CAD build for the part. Positions are in the model's coordinates, mm. Face numbers are marked on the shaded views. Give positions to 0.01 mm unless a question says otherwise; leave off trailing zeros. Loops run counter-clockwise (first coordinate to the right, second up) from the corner with the lowest first, then second, coordinate; pieces in that order, holes last. Notation, with made-up numbers: (70, 0.5) -> (77, 0.5) arc R21 cw to (77, 30.5) -> close; hole circle Ø3 at (13, 13). An arc over 180 degrees is marked (long way). Use one line per item in the form item = value.
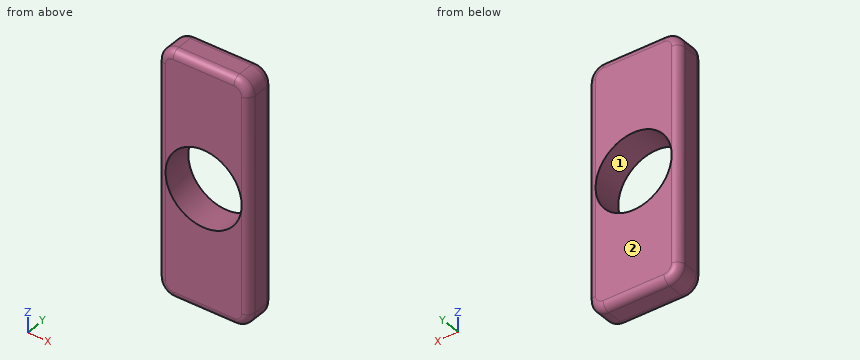
```python
from build123d import *

# Parameters (mm, degrees)
F0_W     = 30
F0_H     = 80
F1_DEPTH = 10
F2_R     = 5
F3_R     = 5
F4_R     = 5
F5_R     = 5
F6_R     = 2.5
F7_R     = 2.5
F9_D     = 25


with BuildPart() as f1:
    # F0 (on Front) → F1 (new body)
    with BuildSketch(Plane.XZ):
        with Locations((15, 40)):
            Rectangle(F0_W, F0_H)
    extrude(amount=F1_DEPTH)

    # F2
    f2_edges = [f1.edges().sort_by_distance(p)[0] for p in [
        (30, -5, 80),
    ]]
    fillet(f2_edges, radius=F2_R)

    # F3
    f3_edges = [f1.edges().sort_by_distance(p)[0] for p in [
        (0, -5, 80),
    ]]
    fillet(f3_edges, radius=F3_R)

    # F4
    f4_edges = [f1.edges().sort_by_distance(p)[0] for p in [
        (0, -5, 0),
    ]]
    fillet(f4_edges, radius=F4_R)

    # F5
    f5_edges = [f1.edges().sort_by_distance(p)[0] for p in [
        (30, -5, 0),
    ]]
    fillet(f5_edges, radius=F5_R)

    # F6
    f6_edges = [f1.edges().sort_by_distance(p)[0] for p in [
        (28.535534, -10, 78.535534),
    ]]
    fillet(f6_edges, radius=F6_R)

    # F7
    f7_edges = [f1.edges().sort_by_distance(p)[0] for p in [
        (28.535534, 0, 78.535534),
    ]]
    fillet(f7_edges, radius=F7_R)

    # F9 (through all)
    with Locations(Plane.XZ.offset(10)):
        with Locations((15, 40)):
            Hole(F9_D / 2)


solid = f1.part
```
1. Drop a flat-ended pin along its axis: P1, Ø1, axis at x = 11, y = -9, coming from the +Z side. Give the stop position or say it passes through.
Result sheet:
P1 = 79.79
2. Cut at B-B, the plane x = 15. Write the cut outline in (y, z).
Result sheet:
outline = (-10, 2.5) arc R2.5 ccw to (-7.5, 0) -> (-2.5, 0) arc R2.5 ccw to (0, 2.5) -> (0, 27.5) -> (-10, 27.5) -> close; (-10, 52.5) -> (0, 52.5) -> (0, 77.5) arc R2.5 ccw to (-2.5, 80) -> (-7.5, 80) arc R2.5 ccw to (-10, 77.5) -> close
3. Cut at D-D, the plane z = 33.5. Write the cut outline in (x, y), then the cut area to 3 significant figures.
Result sheet:
outline = (0, -7.5) arc R2.5 ccw to (2.5, -10) -> (4.32, -10) -> (4.32, 0) -> (2.5, 0) arc R2.5 ccw to (0, -2.5) -> close; (25.68, -10) -> (27.5, -10) arc R2.5 ccw to (30, -7.5) -> (30, -2.5) arc R2.5 ccw to (27.5, 0) -> (25.68, 0) -> close
area = 81.1 mm^2
4. Cut at C-C, the plane z = 58. Write the cut outline in (x, y).
Result sheet:
outline = (0, -7.5) arc R2.5 ccw to (2.5, -10) -> (27.5, -10) arc R2.5 ccw to (30, -7.5) -> (30, -2.5) arc R2.5 ccw to (27.5, 0) -> (2.5, 0) arc R2.5 ccw to (0, -2.5) -> close
5. Drill centre lines: line 1 (Z direction, x = 15, y = -4.25); line 2 (X direction, y = -3.5, z = 40); line 3 (Z direction, x = 23.5, y = -0.75). Where is each one in solid material? Low to high.
Result sheet:
line_1 = 0 to 27.5, 52.5 to 80
line_2 = 0 to 2.5, 27.5 to 30
line_3 = 0.71 to 30.83, 49.17 to 79.29
6. Mould opens along X. For the marked faces 1 and 2 say: pulls with the +X half, pulls with the -X half, needs draft (parallel to the pull), parting line crosses it, or undercut.
Result sheet:
face_1 = undercut
face_2 = needs draft
7. Cut at A-A, the plane y = -5. Write the cut outline in (x, z).
Result sheet:
outline = (0, 5) arc R5 ccw to (5, 0) -> (25, 0) arc R5 ccw to (30, 5) -> (30, 75) arc R5 ccw to (25, 80) -> (5, 80) arc R5 ccw to (0, 75) -> close; hole circle Ø25 at (15, 40)
